from build123d import *

# Parameters (mm, degrees)
SKETCH1_W               = 101.6
SKETCH1_H               = 101.6
BOSS_EXTRUDE1_DEPTH     = 914.4
CUT_EXTRUDE1_DEPTH      = 922.428543079
CUT_EXTRUDE1_DEPTH_BACK = 922.428543079
SKETCH2_W               = 101.6
SKETCH2_H               = 50.8
SKETCH3_W               = 50.8
SKETCH3_H               = 101.6
CUT_EXTRUDE2_DEPTH      = 50.8
SKETCH4_W               = 50.8
SKETCH4_H               = 25.4
CUT_EXTRUDE3_DEPTH      = 50.8
SKETCH5_W               = 76.2
SKETCH5_H               = 50.8
CUT_EXTRUDE4_DEPTH      = 922.428543079


with BuildPart() as part:
    # Sketch1 → Boss-Extrude1 (new body)
    with BuildSketch(Plane.XY):
        Rectangle(SKETCH1_W, SKETCH1_H)
    extrude(amount=BOSS_EXTRUDE1_DEPTH)

    # Sketch2 → Cut-Extrude1 (cut, two sides: drawn at the far end of the back side and taken through both)
    with BuildSketch(Plane(origin=(50.8, 0, 0), x_dir=(0, 0, -1), z_dir=(1, 0, 0)).offset(-CUT_EXTRUDE1_DEPTH_BACK)):
        with Locations((-152.4, 0)):
            Rectangle(SKETCH2_W, SKETCH2_H)
    extrude(amount=CUT_EXTRUDE1_DEPTH + CUT_EXTRUDE1_DEPTH_BACK, mode=Mode.SUBTRACT)

    # Sketch3 → Cut-Extrude2 (cut)
    with BuildSketch(Plane.XY.offset(914.4)):
        Rectangle(SKETCH3_W, SKETCH3_H)
    extrude(amount=-CUT_EXTRUDE2_DEPTH, mode=Mode.SUBTRACT)

    # Sketch4 → Cut-Extrude3 (cut)
    with BuildSketch(Plane.XY.offset(863.6)):
        with Locations((0, 38.1)):
            Rectangle(SKETCH4_W, SKETCH4_H)
        with Locations((0, -38.1)):
            Rectangle(SKETCH4_W, SKETCH4_H)
    extrude(amount=-CUT_EXTRUDE3_DEPTH, mode=Mode.SUBTRACT)

    # Sketch5 → Cut-Extrude4 (cut, through all)
    with BuildSketch(Plane.ZY.offset(50.8)):
        with Locations((381, 0)):
            Rectangle(SKETCH5_W, SKETCH5_H)
    extrude(amount=-CUT_EXTRUDE4_DEPTH, mode=Mode.SUBTRACT)


solid = part.part
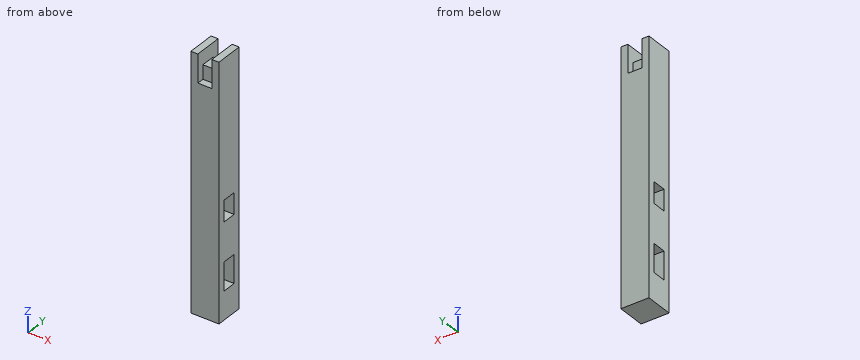
Source: CAD feature listing. Evaluate the final solid. Frame: model axes, mm. Coordinates: 2 decimals unless noted, no trailing zeros. Loops run counter-clockwise (first coordinate to the right, second up) from the corner with the lowest first, then second, coordinate; pieces in that order, holes last. Notation, with made-up numbers: M -32.5,34 L -28.5,34 A26 cw -28.5,55 Z; hole C -2.75,87.25 d4. An arc over 180 degrees is marked long. Answer in a Markdown table with one row per item.
Q1. Section D-D on y = -40. Return the cut outline in (x, z), plus the area to 3 significant figures.
Answers below:
| item | result |
|---|---|
| outline | M -50.8,0 L 50.8,0 L 50.8,914.4 L 25.4,914.4 L 25.4,812.8 L -25.4,812.8 L -25.4,914.4 L -50.8,914.4 Z |
| area | 87,700 mm^2 |
Q2. Section A-A on y = -2. Return the cut outline in (x, z).
Answers below:
| item | result |
|---|---|
| outline | M -50.8,0 L 50.8,0 L 50.8,101.6 L -50.8,101.6 Z; M -50.8,203.2 L 50.8,203.2 L 50.8,342.9 L -50.8,342.9 Z; M -50.8,419.1 L 50.8,419.1 L 50.8,914.4 L 25.4,914.4 L 25.4,863.6 L -25.4,863.6 L -25.4,914.4 L -50.8,914.4 Z |
Q3. Ray query, probe 1 along Z at (x, y) = (38.5, -4.5); probe 2 along Z at (x, y) = (19.5, -14.5); probe 3 along X at (y, z) = (-37, 845). Return the intervals inside material, ascending. Write a range as from..to.
Answers below:
| item | result |
|---|---|
| probe 1 | z = 0..101.6, 203.2..342.9, 419.1..914.4 |
| probe 2 | z = 0..101.6, 203.2..342.9, 419.1..863.6 |
| probe 3 | x = -50.8..-25.4, 25.4..50.8 |
Q4. Section C-C on z = 369. Return the cut outline in (x, y), plus the area to 3 significant figures.
Answers below:
| item | result |
|---|---|
| outline | M -50.8,-50.8 L 50.8,-50.8 L 50.8,-25.4 L -50.8,-25.4 Z; M -50.8,25.4 L 50.8,25.4 L 50.8,50.8 L -50.8,50.8 Z |
| area | 5,160 mm^2 |
Q5. First-contact query: pin 1 (6 mm diameter, centred on x = 20.5, y = -16.5, fed in from +Z); pin 2 (2 mm diameter, centred on x = -20, y = 39.5, fed in from +Z); pin 3 (15 mm diameter, centred on x = -10, z = 829.5, fed in from +Y). Flat tips, straight axial feed; report the tip coordinate or a pass-through.
Answers below:
| item | result |
|---|---|
| pin 1 | stops at z = 863.6 |
| pin 2 | stops at z = 812.8 |
| pin 3 | stops at y = 25.4 |
Q6. Section B-B on x = -9. Return the cut outline in (y, z).
Answers below:
| item | result |
|---|---|
| outline | M -50.8,0 L 50.8,0 L 50.8,812.8 L 25.4,812.8 L 25.4,863.6 L -25.4,863.6 L -25.4,812.8 L -50.8,812.8 Z; hole M -25.4,101.6 L 25.4,101.6 L 25.4,203.2 L -25.4,203.2 Z; hole M -25.4,342.9 L 25.4,342.9 L 25.4,419.1 L -25.4,419.1 Z |
